from build123d import *

# Parameters (mm, degrees)
SKETCH043_W     = 514
SKETCH043_H     = 410
PAD016_DEPTH    = 18
SKETCH044_W     = 514
SKETCH044_H     = 18
POCKET027_DEPTH = 12
SKETCH045_R     = 2.25
POCKET028_DEPTH = 18


with BuildPart() as part:
    # Sketch043 → Pad016 (new body)
    with BuildSketch(Plane.XY):
        with Locations((0, 205)):
            Rectangle(SKETCH043_W, SKETCH043_H)
    extrude(amount=PAD016_DEPTH)

    # Sketch044 (on Face6 of Pad016) → Pocket027 (cut)
    with BuildSketch(Plane.XY.offset(18)):
        with Locations((0, 401)):
            Rectangle(SKETCH044_W, SKETCH044_H)
    extrude(amount=-POCKET027_DEPTH, mode=Mode.SUBTRACT)

    # Sketch045 (on Face7 of Pocket027) → Pocket028 (cut)
    with BuildSketch(Plane.XY.offset(18)):
        with Locations((-221, 24)):
            Circle(SKETCH045_R)
        with Locations((-221, 368)):
            Circle(SKETCH045_R)
    pocket028 = extrude(amount=-POCKET028_DEPTH, mode=Mode.SUBTRACT)

    # Mirrored010: Pocket028 across Sketch045 V_Axis
    add(pocket028.mirror(Plane(origin=(0, 0, 18), x_dir=(0, 0, 1), z_dir=(1, 0, 0))), mode=Mode.SUBTRACT)


solid = part.part
Here's how the part is built. I have some questions about the finished solid (model axes, mm). A direction names the side the tool comes from. Round coordinates to 2 decimals unless told otherwise and drop trailing zeros. Loops run counter-clockwise (first coordinate to the right, second up) from the corner with the lowest first, then second, coordinate; pieces in that order, holes last.
1. If we section it at A-A on z = 8.75: Write out the boundary of the cut face in (x, y), plus the area to 3 significant figures.
Answer list:
outline: (-257, 0) - (257, 0) - (257, 392) - (-257, 392) - close; hole circle Ø4.5 at (-221, 24); hole circle Ø4.5 at (-221, 368); hole circle Ø4.5 at (221, 24); hole circle Ø4.5 at (221, 368)
area: 201,000 mm2
2. Which directions (+Z, -Z, +X, -X, +Y, -Y) give clear straight access to the entire face, cutting with the end or side of a thin tool? Please do faces 1 (the face through (-4, 392, 12)), 2 (the face through (-4, 199, 18)).
Answer list:
face 1: +Z, +X, -X, +Y
face 2: +Z, +X, -X, +Y, -Y
3. If I drill on line 1 along Y through (x, z) = (-221, 13.25); line 2 along Y through (x, z) = (-221, 4); line 3 along X through (y, z) = (368, 4.25), over which ranges is the centre line in solid material (lowest first)?
Answer list:
line 1: y = 0 to 21.75, 26.25 to 365.75, 370.25 to 392
line 2: y = 0 to 21.75, 26.25 to 365.75, 370.25 to 410
line 3: x = -257 to -223.25, -218.75 to 218.75, 223.25 to 257
4. For P1, Ø5.5, axis at x = -118.5, y = 403, coming from the +Z side; P2, Ø3.5, axis at x = -221, y = 24, coming from the -Z side; P3, Ø1, axis at x = -121, z = 14, coming from the +Y side, each with a flat end and sliding along its axis, tell me the tip position at first contact or that it passes through.
Answer list:
P1: stops at z = 6
P2: passes through
P3: stops at y = 392
5. If we section it at B-B on x = 31.5: Write out the boundary of the cut face in (y, z).
Answer list:
outline: (0, 0) - (410, 0) - (410, 6) - (392, 6) - (392, 18) - (0, 18) - close
